Source: three-view drawing plus pictorial views. Frame: mm from the lowest corner of the part. A direction names the side the tool comes from. Coordinates: 2 decimals unless noted, no trailing zeros. Write each loop counter-clockwise with the first axis right and the second up, starting at its lowest first coordinate (ties: lowest second). Pieces come first, ordered by that corner, then holes. Notation, with made-up numbers: (56, 69) - (66, 69) arc R24 cw to (66, 100) - close; hole circle Ø9 at (-25, 56.25). An arc over 180 degrees is marked (long way). Put each result on its own line as item: value. Start each with the question number.
1. Cut plane D-D, the plane z = 180. Return loops of the section in (x, y).
2. Access query for the marked faces 4 and 5. Directions: +Z, -Z, +X, -X, +Y, -Y. A direction counts if a zero-diameter tool reaches every point of the face in a straight line with its end or side. Return the directions, or none.
3. Line query: line 1 (Y direction, x = 19, z = 61); line 2 (Z direction, x = 100, y = 504); line 3 (X direction, y = 354.5, z = 97.5). Output: solid intervals per line, ascending.
4. Cut plane A-A, the plane x = 180. Return loops of the section in (y, z).
5. Pin query (flat end, axial travel): pin 1 (14.5 mm diameter, centred on x = 180, z = 100, fed in from +Y); pin 2 (1 mm diameter, centred on y = 206.5, z = 74.5, fed in from -X); pin 3 (10 mm diameter, centred on y = 305.5, z = 118.5, fed in from -X); pin 4 (6 mm diameter, centred on y = 250, z = 59.5, fed in from -X). Return the tip coordinate at first contact, or that it passes through.
6. Cut plane B-B, the plane z = 100. Count the separate pieces of the cut face and the enclosed holes in it, and give its area (3 significant figures).
7. Pull-direction query (Z, two-part tool) for the marked faces 1, 2 and 3; classes: released by +Z, released by -Z, zero draft, split by the parting line, or undercut.
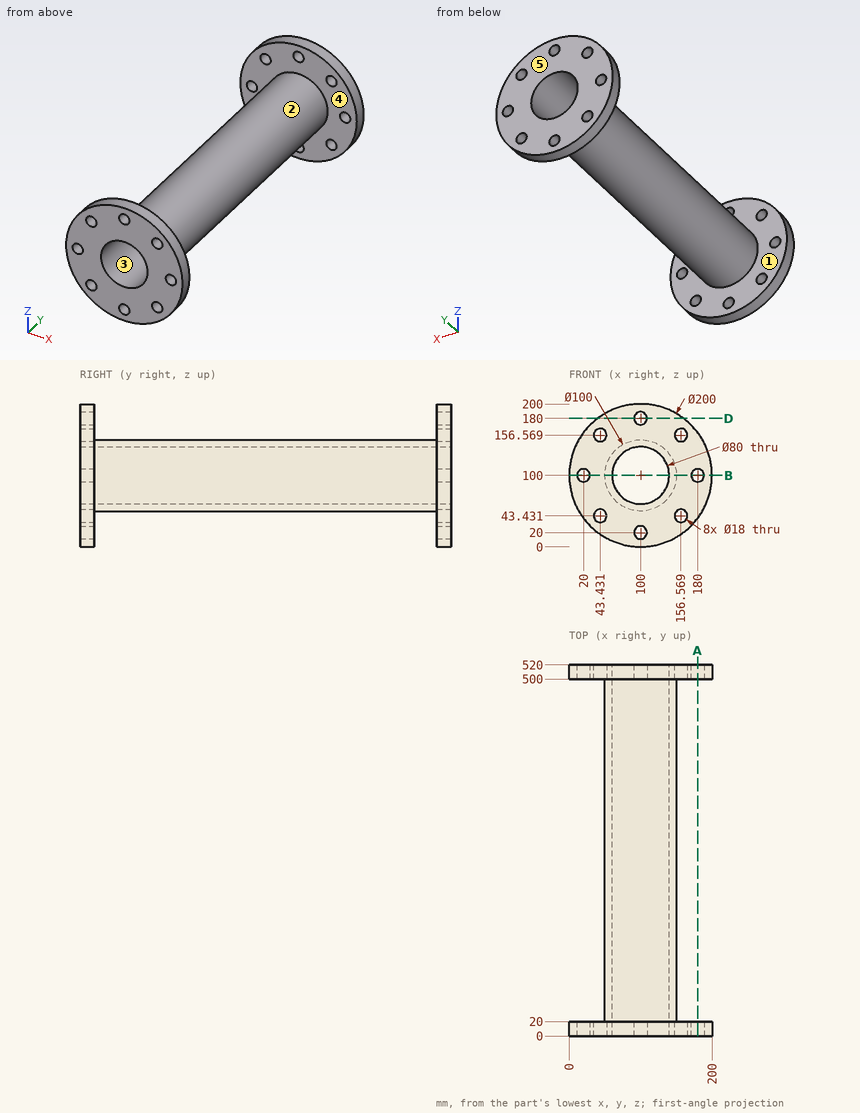
Report:
1. outline: (40, 0) - (91, 0) - (91, 20) - (40, 20) - close; (40, 500) - (91, 500) - (91, 520) - (40, 520) - close; (109, 0) - (160, 0) - (160, 20) - (109, 20) - close; (109, 500) - (160, 500) - (160, 520) - (109, 520) - close
2. face 4: none
2. face 5: +Z, -Z, +X, -X, +Y
3. line 1: y = 0 to 20, 500 to 520
3. line 2: z = 0 to 11, 29 to 60, 140 to 171, 189 to 200
3. line 3: x = 50.06 to 60.08, 139.92 to 149.94
4. outline: (0, 40) - (20, 40) - (20, 91) - (0, 91) - close; (0, 109) - (20, 109) - (20, 160) - (0, 160) - close; (500, 40) - (520, 40) - (520, 91) - (500, 91) - close; (500, 109) - (520, 109) - (520, 160) - (500, 160) - close
5. pin 1: passes through
5. pin 2: stops at x = 56.7
5. pin 3: stops at x = 51.86
5. pin 4: stops at x = 66.93
6. separate pieces: 6
6. enclosed holes: 0
6. area: 13,000 mm^2
7. face 1: zero draft
7. face 2: split by the parting line
7. face 3: undercut
